Here's how the part is built. I have some questions about the finished solid (model axes, mm). A direction names the side the tool comes from. Round coordinates to 2 decimals unless told otherwise and drop trailing zeros. Write each loop counter-clockwise with the first axis right and the second up, starting at its lowest first coordinate (ties: lowest second). Pieces come first, ordered by that corner, then holes. Notation, with made-up numbers: M -20.5,18.5 L 18.5,18.5 A22 cw 18.5,46.5 Z; hole C 69.5,85.25 d10. An arc over 180 degrees is marked long. Write item = value, one per line. Start each with the question number.
(1) I want a section at B-B (y = 37). List the corners of the cut face in (x, z) for me.
(2) On a 3-axis mill with a long thin cutter (end or side, diameter ignored), from which of +Z, -Z, +X, -X, +Y, -Y can I reach the whole of each face in a straight line? I mean faces 1 (the flat face through (-9, 54.798, 2)), 2 (the flat face through (39.347, 12, -7)), 3 (the flat face through (-45.653, 12, -7)). Say none if no direction works.
(3) Will these pins go through, and if not, where does the flat tip stop? pin 1 Ø6 at (x, y) = (39.58, -29.44) entering from -Z; pin 2 Ø1.5 at (x, z) = (15.5, -12) entering from -Y; pin 3 Ø12 at (y, z) = (18.5, -11) entering from +X.
(4) I want a section at A-A (x = -7.5). List the corners of the cut face in (y, z) for me, and give its area (3 significant figures).
(5) I want a section at C-C (z = -3.5). List the corners of the cut face in (x, y) for me, and give its area (4 significant figures).
(6) If we mould it in two halves opening along Y, with no side actions, what happens to faces 4 (the flat face through (-4, 39.798, -7)), 5 (the flat face through (-4, -15.202, -7)), 6 (the cylindrical face through (39.895, 52.396, 2.465))? For each: released by +Y, released by -Y, zero draft, split by the parting line, or undercut.
(7) I want a section at D-D (x = 20). List the corners of the cut face in (y, z) for me, and give its area (3 significant figures).
(8) I need wall thicknesses on line 1 along X through (y, z) = (51, 2.25); line 2 along Y through (x, z) = (-15.5, -4.25); line 3 along Z through (x, y) = (-10, -17.5). Which ranges of each line are inside material? Lowest first, please.
```python
from build123d import *

# Parameters (mm, degrees)
F0_W     = 105
F0_H     = 89
F2_DEPTH = 5
F1_W     = 85
F1_H     = 55
F3_DEPTH = 15
F4_W     = 19.05
F4_H     = 15.24
F5_DEPTH = 1.27
F7_D     = 4.7625


with BuildPart() as f2:
    # F0 (on Top) → F2 (new body)
    with BuildSketch(Plane.XY):
        with Locations((-8.15268, 10.297881)):
            Rectangle(F0_W, F0_H)
    extrude(amount=F2_DEPTH)

    # F1 (on face) → F3 (join)
    with BuildSketch(Plane.XY):
        with Locations((-3.15268, 12.297881)):
            Rectangle(F1_W, F1_H)
    extrude(amount=-F3_DEPTH)

    # F4 (on face) → F5 (join)
    with BuildSketch(Plane.XY.offset(5)):
        with Locations((-34.587345, 7.62)):
            Rectangle(F4_W, F4_H)
        with Locations((-12.761215, 7.62)):
            Rectangle(F4_W, F4_H)
    extrude(amount=F5_DEPTH)

    # F7 (through all)
    with Locations(Plane.XY.offset(5)):
        with Locations((-55.89018, 50.035381), (-55.89018, -29.439619), (39.58482, 50.035381), (39.58482, -29.439619)):
            Hole(F7_D / 2)


solid = f2.part
```
Returned:
q1.outline = M -60.65,0 L -45.65,0 L -45.65,-15 L 39.35,-15 L 39.35,0 L 44.35,0 L 44.35,5 L -60.65,5 Z
q2.face_1 = +Z, -Z, +X, -X, +Y
q2.face_2 = -Z, +X, +Y, -Y
q2.face_3 = -Z, -X, +Y, -Y
q3.pin_1 = 0
q3.pin_2 = -15.2
q3.pin_3 = 39.35
q4.outline = M -34.2,0 L -15.2,0 L -15.2,-15 L 39.8,-15 L 39.8,0 L 54.8,0 L 54.8,5 L 15.24,5 L 15.24,6.27 L 0,6.27 L 0,5 L -34.2,5 Z
q4.area = 1,290 mm²
q5.outline = M -45.65,-15.2 L 39.35,-15.2 L 39.35,39.8 L -45.65,39.8 Z
q5.area = 4,675 mm²
q6.face_4 = released by +Y
q6.face_5 = released by -Y
q6.face_6 = undercut
q7.outline = M -34.2,0 L -15.2,0 L -15.2,-15 L 39.8,-15 L 39.8,0 L 54.8,0 L 54.8,5 L -34.2,5 Z
q7.area = 1,270 mm²
q8.line_1 = -60.65 to -58.07, -53.71 to 37.41, 41.76 to 44.35
q8.line_2 = -15.2 to 39.8
q8.line_3 = 0 to 5
